Read the model definition and answer for the solid it produces. Units are mm, in the model's axes. A direction names the side the tool comes from. Coordinates: 2 decimals unless noted, no trailing zeros. Loops run counter-clockwise (first coordinate to the right, second up) from the corner with the lowest first, then second, coordinate; pieces in that order, holes last. Notation, with made-up numbers: M 87,-20.5 L 99,-20.5 A9 ccw 99,-8.5 Z; hole C 70,63 d2. An arc over 180 degrees is marked long. Use one line per item in the form item = value. Start each with the question number.
1. A tool of negligible diameter and unlimited length cuts with its end or side. For faces 5 (the flat face through (-1, 62, -82.55)), 6 (the flat face through (-74, 25, 58)), from which of +Z, -Z, +X, -X, +Y, -Y can it reach the whole face along a straight path? Write none if from no direction.
2. Flat-ended cylindrical pins translate along their axes: pin 1 (10 mm diameter, centred on x = -19, y = 90, fed in from +Z); pin 2 (5 mm diameter, centred on x = -68.5, z = 14.5, fed in from +Y); pin 3 (2 mm diameter, centred on x = 40.5, z = -60.5, fed in from +Y). Find the tip coordinate at first contact, or state that the pin passes through.
3. The part is cut by section B-B (z = -71.5). Give the vertices of the cut face in (x, y).
4. For a pull along X with two mould halves and no side action, classify faces 1 (the flat face through (82.55, 43, -1)), 2 (the flat face through (-12, -4, 78.74)), 3 (the flat face through (-1, -38.1, -1)), 4 (the flat face through (0, 127, -80)) as released by +X, released by -X, zero draft, split by the parting line, or undercut.
5. The part is cut by section D-D (z = -41.5). Give the vertices of the cut face in (x, y).
6. Find the intervals of material crossed by probe 1 along X at (y, z) = (35, 68); probe 2 along X at (y, z) = (14.5, -4); probe 3 along Y at (x, z) = (-12, 57), in increasing order. Write a range as [from, to].
7. The part is cut by section C-C (y = 115). Give the vertices of the cut face in (x, z), plus the area to 3 significant figures.
8. The part is cut by section A-A (x = 29). Give the vertices of the cut face in (y, z).
from build123d import *

# Parameters (mm, degrees)
SKETCH1_W           = 6.35
SKETCH1_H           = 129.54
BOSS_EXTRUDE1_DEPTH = 127
BOSS_EXTRUDE2_DEPTH = 38.1
SKETCH5_W           = 165.1
SKETCH5_H           = 165.1
BOSS_EXTRUDE3_DEPTH = 5.08
SKETCH6_W           = 139.7
SKETCH6_H           = 127
CUT_EXTRUDE1_DEPTH  = 12.7
SKETCH1_4_W         = 6.35
SKETCH1_4_H         = 129.54
BOSS_EXTRUDE5_DEPTH = 41.656
SKETCH8_W           = 6.35
SKETCH8_H           = 129.54
BOSS_EXTRUDE6_DEPTH = 50.8
CUT_EXTRUDE2_DEPTH  = 166.1


with BuildPart() as part:
    # Sketch1 → Boss-Extrude1 (new body)
    with BuildSketch(Plane(origin=(0, 0, 0), x_dir=(1, 0, 0), z_dir=(0, 1, 0))):
        Polygon((0, 78.74), (0, 82.55), (-82.55, 82.55), (-82.55, -82.55), (0, -82.55), (0, -78.74), (-78.74, -78.74), (-78.74, -64.77), (-78.74, 64.77), (-78.74, 78.74), align=None)
        with Locations((-75.565, 0)):
            Rectangle(SKETCH1_W, SKETCH1_H)
        Polygon((82.55, 82.55), (0, 82.55), (0, 78.74), (78.74, 78.74), (78.74, 64.77), (78.74, -64.77), (78.74, -78.74), (0, -78.74), (0, -82.55), (82.55, -82.55), align=None)
        with Locations((75.565, 0)):
            Rectangle(SKETCH1_W, SKETCH1_H)
    extrude(amount=BOSS_EXTRUDE1_DEPTH)

    # Sketch4 → Boss-Extrude2 (add)
    with BuildSketch(Plane.XZ):
        Polygon((-82.55, 82.55), (-82.55, -82.55), (-78.74, -82.55), (-78.74, -78.74), (-78.74, -64.77), (-78.74, 64.77), (-78.74, 78.74), (78.74, 78.74), (78.74, 64.77), (78.74, -64.77), (78.74, -78.74), (78.74, -82.55), (82.55, -82.55), (82.55, 82.55), align=None)
    extrude(amount=BOSS_EXTRUDE2_DEPTH)

    # Sketch5 → Boss-Extrude3 (add)
    with BuildSketch(Plane.XZ.offset(38.1)):
        Rectangle(SKETCH5_W, SKETCH5_H)
    extrude(amount=BOSS_EXTRUDE3_DEPTH)

    # Sketch6 → Cut-Extrude1 (cut)
    with BuildSketch(Plane.XY.offset(82.55)):
        with Locations((0, 63.5)):
            Rectangle(SKETCH6_W, SKETCH6_H)
    extrude(amount=-CUT_EXTRUDE1_DEPTH, mode=Mode.SUBTRACT)

    # Sketch1_4 → Boss-Extrude5 (add)
    with BuildSketch(Plane(origin=(0, 0, 0), x_dir=(1, 0, 0), z_dir=(0, 1, 0))):
        with Locations((75.565, 0)):
            Rectangle(SKETCH1_4_W, SKETCH1_4_H)
        with Locations((-75.565, 0)):
            Rectangle(SKETCH1_4_W, SKETCH1_4_H)
    extrude(amount=-BOSS_EXTRUDE5_DEPTH)

    # Sketch8 → Boss-Extrude6 (add)
    with BuildSketch(Plane(origin=(0, -38.1, 0), x_dir=(1, 0, 0), z_dir=(0, 1, 0))):
        with Locations((-69.215, 0)):
            Rectangle(SKETCH8_W, SKETCH8_H)
        with Locations((69.215, 0)):
            Rectangle(SKETCH8_W, SKETCH8_H)
    extrude(amount=BOSS_EXTRUDE6_DEPTH)

    # Sketch9 → Cut-Extrude2 (cut, through all)
    with BuildSketch(Plane(origin=(0, -38.1, 0), x_dir=(1, 0, 0), z_dir=(0, 1, 0))):
        Polygon((-78.74, 64.77), (-66.04, 46.632520314), (-66.04, 64.77), align=None)
        Polygon((-78.74, -64.77), (-66.04, -64.77), (-66.04, -46.632520314), align=None)
        Polygon((78.74, -64.77), (66.04, -64.77), (66.04, -46.632520314), align=None)
        Polygon((66.04, 64.77), (66.04, 46.632520314), (78.74, 64.77), align=None)
    extrude(amount=CUT_EXTRUDE2_DEPTH, mode=Mode.SUBTRACT)


solid = part.part
Computed values:
q1.face_5 = -Z, +X, -X, +Y, -Y
q1.face_6 = +Y
q2.pin_1 = -78.74
q2.pin_2 = 12.7
q2.pin_3 = -38.1
q3.outline = M -82.55,-43.18 L 82.55,-43.18 L 82.55,127 L 78.74,127 L 78.74,-38.1 L -78.74,-38.1 L -78.74,127 L -82.55,127 Z
q4.face_1 = released by +X
q4.face_2 = undercut
q4.face_3 = undercut
q4.face_4 = zero draft
q5.outline = M -82.55,-43.18 L 82.55,-43.18 L 82.55,127 L 72.39,127 L 72.39,12.7 L 66.04,12.7 L 66.04,-38.1 L -66.04,-38.1 L -66.04,12.7 L -72.39,12.7 L -72.39,127 L -82.55,127 Z
q6.probe_1 = [-82.55, -78.74], [78.74, 82.55]
q6.probe_2 = [-82.55, -72.39], [72.39, 82.55]
q6.probe_3 = [-43.18, -38.1]
q7.outline = M -82.55,-82.55 L 82.55,-82.55 L 82.55,82.55 L 69.85,82.55 L 69.85,78.74 L 78.74,78.74 L 78.74,64.77 L 72.39,55.7 L 72.39,-55.7 L 78.74,-64.77 L 78.74,-78.74 L -78.74,-78.74 L -78.74,-64.77 L -72.39,-55.7 L -72.39,55.7 L -78.74,64.77 L -78.74,78.74 L -69.85,78.74 L -69.85,82.55 L -82.55,82.55 Z
q7.area = 3,460 mm²
q8.outline = M -43.18,-82.55 L -38.1,-82.55 L -38.1,78.74 L 0,78.74 L 0,82.55 L -43.18,82.55 Z; M 0,-82.55 L 127,-82.55 L 127,-78.74 L 0,-78.74 Z
